Model file for the job. Use its own axes, mm. Face numbers are marked on the shaded views. Round coordinates to 2 decimals unless told otherwise and drop trailing zeros. Loops run counter-clockwise (first coordinate to the right, second up) from the corner with the lowest first, then second, coordinate; pieces in that order, holes last. Notation, with made-up numbers: M -23,35 L 14,35 A10 cw 14,41 Z; hole C 8,29 d4. An arc over 180 degrees is marked long. Use a Markdown table: item, result. Add a question column.
Q1. Probe line 1 (X direction, y = 0, z = 0.95); line 2 (X direction, y = -0.25, z = 2); line 3 (Y direction, x = -28, z = 0.95). List the from-to ranges inside material, lowest first. Write a range as from..to.
Q2. Mould opens along Y. For the marked faces 1 and 2 say: +Y half, -Y half, draft (parallel to the pull), parting line (faces both ways), or undercut.
Q3. Pin check, flat tips, straight feed: pin 1 (4 mm diameter, centred on x = 28, y = 0, fed in from -Z); pin 2 (4 mm diameter, centred on x = 0, y = -4, fed in from +Z). Stop position of each tip, or through.
Q4. Cut at D-D (x = 5). Give the cut face in (y, z).
Q5. Cut at B-B (y = 0). Give the cut face in (x, z).
Q6. Cut at C-C (z = 1.4). Give the cut face in (x, y), plus the area to 3 significant figures.
Q7. Cut at A-A (x = 28). Give the cut face in (y, z).
from build123d import *

# Parameters (mm, degrees)
CYLINDER002_R     = 2.1
CYLINDER002_DEPTH = 10
CYLINDER001_R     = 2.1
CYLINDER001_DEPTH = 10
BOX012_W          = 40
BOX012_H          = 16
BOX012_DEPTH      = 2.5
BOX011_W          = 76
BOX011_H          = 20
BOX011_DEPTH      = 2.5
FILLET014_R       = 3


with BuildPart() as cylinder002:
    # Cylinder002 → Cylinder002 (new body)
    with BuildSketch(Plane(origin=(28, 0, -2), x_dir=(1, 0, 0), z_dir=(0, 0, 1))):
        Circle(CYLINDER002_R)
    extrude(amount=CYLINDER002_DEPTH)


with BuildPart() as fusion005:
    # Cylinder001 → Cylinder001 (new body)
    with BuildSketch(Plane(origin=(-28, 0, -2), x_dir=(1, 0, 0), z_dir=(0, 0, 1))):
        Circle(CYLINDER001_R)
    extrude(amount=CYLINDER001_DEPTH)

    # Fusion005: union Cylinder002
    add(cylinder002.part)


with BuildPart() as cube012:
    # Box012 → Box012 (new body)
    with BuildSketch(Plane(origin=(-20, -8, 1), x_dir=(1, 0, 0), z_dir=(0, 0, 1))):
        with Locations((20, 8)):
            Rectangle(BOX012_W, BOX012_H)
    extrude(amount=BOX012_DEPTH)


with BuildPart() as cut017:
    # Box011 → Box011 (new body)
    with BuildSketch(Plane(origin=(-38, -10, 0), x_dir=(1, 0, 0), z_dir=(0, 0, 1))):
        with Locations((38, 10)):
            Rectangle(BOX011_W, BOX011_H)
    extrude(amount=BOX011_DEPTH)

    # Cut016: cut Cube012
    add(cube012.part, mode=Mode.SUBTRACT)

    # Fillet014
    fillet014_edges = [cut017.edges().sort_by_distance(p)[0] for p in [
        (-38, -10, 1.25),
        (-38, 10, 1.25),
        (38, -10, 1.25),
        (38, 10, 1.25),
    ]]
    fillet(fillet014_edges, radius=FILLET014_R)

    # Cut017: cut Fusion005
    add(fusion005.part, mode=Mode.SUBTRACT)


solid = cut017.part
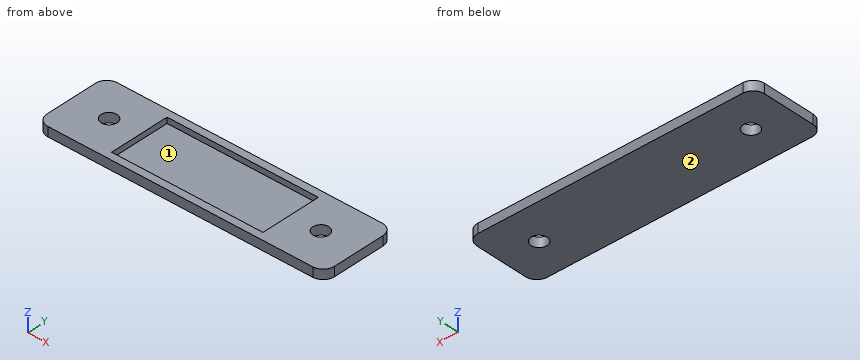
Checked values:
| question | item | result |
|---|---|---|
| 1 | line 1 | x = -38..-30.1, -25.9..25.9, 30.1..38 |
| 1 | line 2 | x = -38..-30.09, -25.91..-20, 20..25.91, 30.09..38 |
| 1 | line 3 | y = -10..-2.1, 2.1..10 |
| 2 | face 1 | undercut |
| 2 | face 2 | draft |
| 3 | pin 1 | passes through |
| 3 | pin 2 | stops at z = 1 |
| 4 | outline | M -10,0 L 10,0 L 10,2.5 L 8,2.5 L 8,1 L -8,1 L -8,2.5 L -10,2.5 Z |
| 5 | outline | M -38,0 L -30.1,0 L -30.1,2.5 L -38,2.5 Z; M -25.9,0 L 25.9,0 L 25.9,2.5 L 20,2.5 L 20,1 L -20,1 L -20,2.5 L -25.9,2.5 Z; M 30.1,0 L 38,0 L 38,2.5 L 30.1,2.5 Z |
| 6 | outline | M -38,-7 A3 ccw -35,-10 L 35,-10 A3 ccw 38,-7 L 38,7 A3 ccw 35,10 L -35,10 A3 ccw -38,7 Z; hole C -28,0 d4.2; hole M -20,-8 L 20,-8 L 20,8 L -20,8 Z; hole C 28,0 d4.2 |
| 6 | area | 845 mm^2 |
| 7 | outline | M -10,0 L -2.1,0 L -2.1,2.5 L -10,2.5 Z; M 2.1,0 L 10,0 L 10,2.5 L 2.1,2.5 Z |
